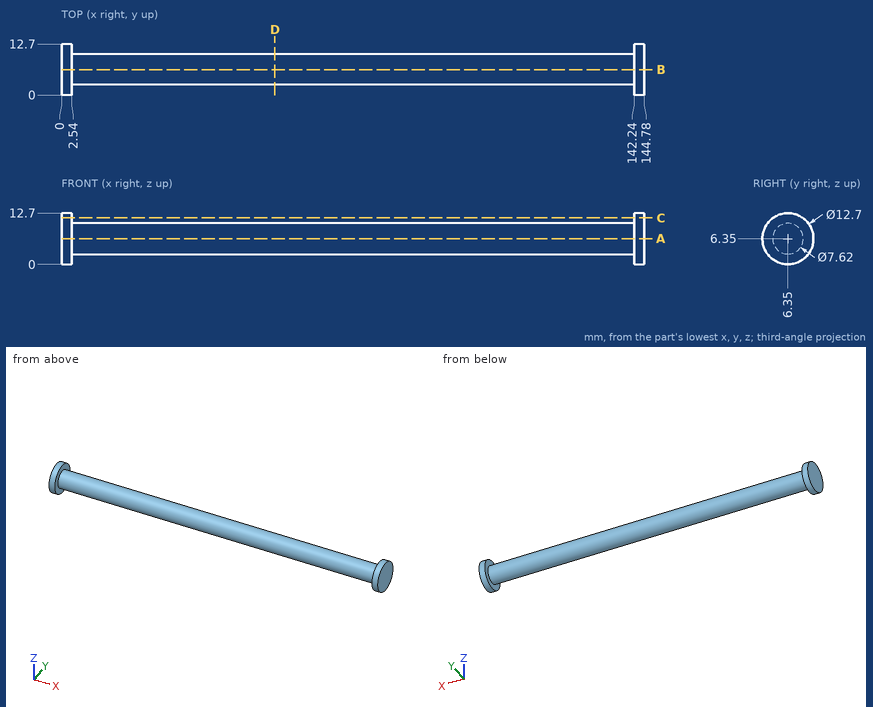
Job drawing, mm, ordinate dimensions from the low corner. One solid piece. Round coordinates to 2 decimals unless told otherwise and drop trailing zeros. Write each loop counter-clockwise with the first axis right and the second up, starting at its lowest first coordinate (ties: lowest second). Pieces come first, ordered by that corner, then holes. Notation, with made-up numbers: M 52.5,75.25 L 63.5,75.25 A22 ccw 63.5,98.25 Z; hole C -7,58 d8. An arc over 180 degrees is marked long. Return JSON: item names as keys, results as strings. Group by question number.
(1) Saw through at D-D on x = 53. Write the cut outline in (y, z).
(2) Saw through at A-A on z = 6.35. Write the cut outline in (x, y).
(3) Drill centre lines: probe 1 along X at (y, z) = (0.5, 5.25); probe 2 along Z at (x, y) = (45, 6.5). Where is each one in solid material? Low to high.
(4) Pin check, flat tips, straight feed: pin 1 Ø5 at (x, y) = (32, 7.5) entering from -Z; pin 2 Ø3 at (x, y) = (127.5, 4) entering from +Z. Stop position of each tip, or through.
(5) Saw through at C-C on z = 11.5. Write the cut outline in (x, y).
Returned:
{
 "1": {"outline": "C 6.35,6.35 d7.62"},
 "2": {"outline": "M 0,0 L 2.54,0 L 2.54,2.54 L 142.24,2.54 L 142.24,0 L 144.78,0 L 144.78,12.7 L 142.24,12.7 L 142.24,10.16 L 2.54,10.16 L 2.54,12.7 L 0,12.7 Z"},
 "3": {"probe 1": "0 to 2.54, 142.24 to 144.78", "probe 2": "2.54 to 10.16"},
 "4": {"pin 1": "z = 2.54", "pin 2": "z = 10.06"},
 "5": {"outline": "M 0,2.64 L 2.54,2.64 L 2.54,10.06 L 0,10.06 Z; M 142.24,2.64 L 144.78,2.64 L 144.78,10.06 L 142.24,10.06 Z"}
}
